from build123d import *

# Parameters (mm, degrees)
BOSS_EXTRUDE1_DEPTH = 50.8
SKETCH2_W           = 50.8
SKETCH2_H           = 25.4
BOSS_EXTRUDE2_DEPTH = 499.2
SKETCH3_W           = 25.4
SKETCH3_H           = 50.8
BOSS_EXTRUDE3_DEPTH = 998.4


with BuildPart() as part:
    # Sketch1 → Boss-Extrude1 (new body)
    with BuildSketch(Plane(origin=(0, 0, 0), x_dir=(0, 0, -1), z_dir=(1, 0, 0))):
        Polygon((0, 720), (0, 0), (-620, 0), (-620, 720), (-594.6, 720), (-594.6, 25.4), (-25.4, 25.4), (-25.4, 720), align=None)
    boss_extrude1 = extrude(amount=BOSS_EXTRUDE1_DEPTH)

    # Sketch2 → Boss-Extrude2 (add)
    with BuildSketch(Plane(origin=(50.8, 0, 0), x_dir=(0, 0, -1), z_dir=(1, 0, 0))):
        with Locations((-310, 12.7)):
            Rectangle(SKETCH2_W, SKETCH2_H)
    boss_extrude2 = extrude(amount=BOSS_EXTRUDE2_DEPTH)

    # Mirror1: Boss-Extrude1, Boss-Extrude2 across plane
    add(boss_extrude1.mirror(Plane(origin=(550, 0, 0), x_dir=(0, 0, 1), z_dir=(1, 0, 0))))
    add(boss_extrude2.mirror(Plane(origin=(550, 0, 0), x_dir=(0, 0, 1), z_dir=(1, 0, 0))))

    # Sketch3 → Boss-Extrude3 (add)
    with BuildSketch(Plane(origin=(50.8, 0, 0), x_dir=(0, 0, -1), z_dir=(1, 0, 0))):
        with Locations((-12.7, 444.6)):
            Rectangle(SKETCH3_W, SKETCH3_H)
    extrude(amount=BOSS_EXTRUDE3_DEPTH)


solid = part.part
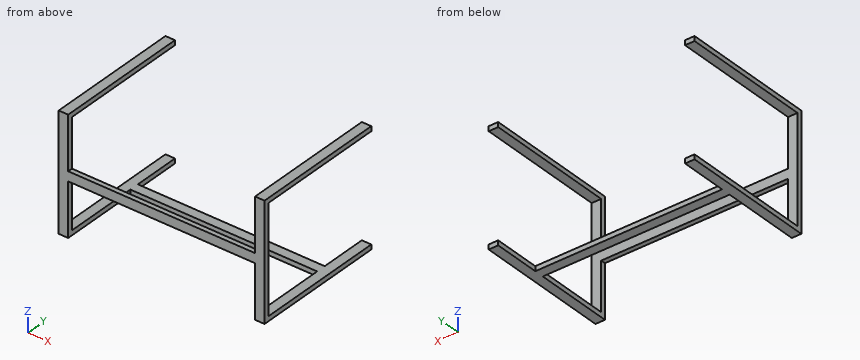
Verification items for the finished model (mm, model axes). Give positions to 0.01 mm unless a question says otherwise; leave off trailing zeros. Loops run counter-clockwise (first coordinate to the right, second up) from the corner with the lowest first, then second, coordinate; pieces in that order, holes last.
1. Cross-section at C-C on y = 173. Record the cut outline in (x, z).
Derived:
outline: (0, 0) - (50.8, 0) - (50.8, 25.4) - (0, 25.4) - close; (0, 594.6) - (50.8, 594.6) - (50.8, 620) - (0, 620) - close; (1049.2, 0) - (1100, 0) - (1100, 25.4) - (1049.2, 25.4) - close; (1049.2, 594.6) - (1100, 594.6) - (1100, 620) - (1049.2, 620) - close
2. Cross-section at A-A on z = 370. Record the cut outline in (x, y), and give its area (3 significant figures).
Derived:
outline: (0, 0) - (50.8, 0) - (50.8, 25.4) - (0, 25.4) - close; (1049.2, 0) - (1100, 0) - (1100, 25.4) - (1049.2, 25.4) - close
area: 2,580 mm2
3. Cross-section at B-B on x = 827. Record the cut outline in (y, z).
Derived:
outline: (0, 284.6) - (25.4, 284.6) - (25.4, 335.4) - (0, 335.4) - close; (419.2, 0) - (470, 0) - (470, 25.4) - (419.2, 25.4) - close
4. Go/stop test with flat-tipped pins: P1, Ø20.5, axis at x = 351, y = 7, coming from the +Z side; P2, Ø5, axis at x = 120, y = 440, coming from the +Z side; P3, Ø7.5, axis at x = 541.5, z = 18.5, coming from the +Y side. Record where each tip stops, or that it passes through.
Derived:
P1: stops at z = 335.4
P2: stops at z = 25.4
P3: stops at y = 470
5. Material ranges on probe 1 along Z at (x, y) = (594, 420), recorded low to high.
Derived:
probe 1: z = 0 to 25.4
